Work out the finished part from the listing and answer in its coordinate system (mm). Face numbers are marked on the shaded views. Round coordinates to 2 decimals unless told otherwise and drop trailing zeros. Write each loop counter-clockwise with the first axis right and the second up, starting at its lowest first coordinate (ties: lowest second). Pieces come first, ordered by that corner, then holes. Notation, with made-up numbers: (-8.75, 42.5) -> (32.25, 42.5) arc R29 cw to (32.25, 77.5) -> close; hole circle Ø2 at (-35, -32.5). An arc over 180 degrees is marked (long way). One line per question, with ' | ' between items. Start each with the question number.
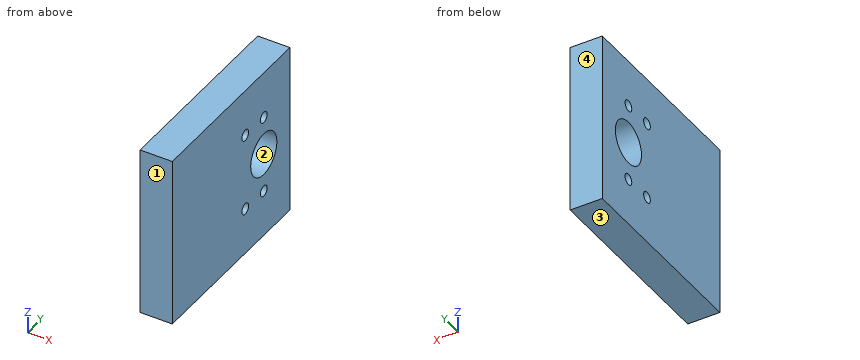
Autodesk Inventor part; units mm, degrees
ref_plane "YZ Plane" through (0, 0, 0) normal (1, 0, 0) x (0, 1, 0)
ref_plane "XZ Plane" through (0, 0, 0) normal (0, 1, 0) x (-1, 0, 0)
ref_plane "XY Plane" through (0, 0, 0) normal (0, 0, 1) x (1, 0, 0)
sketch "Sketch1" plane through (0, 0, 0) normal (1, 0, 0) x (0, 1, 0)
  line L0 (0, 0) -> (114.3, 0)
  line L1 (114.3, 0) -> (114.3, -101.6)
  line L2 (114.3, -101.6) -> (0, -101.6)
  line L3 (0, -101.6) -> (0, 0)
  dimension "d0" = 114.3
  dimension "d1" = 101.6
extrude "Extrusion1" add sketch "Sketch1" along normal blind 19.05
sketch "Sketch2" plane through (19.05, 0, 0) normal (1, 0, 0) x (0, 0, -1)
  circle A0 centre (27.8, 88.9) radius 3.2499
  circle A1 centre (73.8, 88.9) radius 3.2499
  circle A2 centre (73.8, 70.9) radius 3.2499
  circle A3 centre (27.8, 70.9) radius 3.2499
  line L0 (27.8, 88.9) -> (27.8, 70.9)
  line L1 (27.8, 88.9) -> (73.8, 88.9)
  line L2 (27.8, 70.9) -> (73.8, 70.9)
  line L3 (73.8, 70.9) -> (73.8, 88.9)
  line L4 (0, 114.3) -> (0, 0)
  line L5 (101.6, 0) -> (101.6, 114.3)
  line L6 (101.6, 114.3) -> (0, 114.3)
  dimension "d4" = 6.4999
  dimension "d5" = 6.4999
  dimension "d6" = 6.4999
  dimension "d7" = 6.4999
  dimension "d8" = 46
  dimension "d9" = 18
  dimension "d10" = 27.8
  dimension "d11" = 101.6
  dimension "d12" = 25.4
extrude "Extrusion2" cut sketch "Sketch2" against normal blind 19.05 contours L1 L0 A0 | A0 L0 L1 | L1 L3 A1 | A1 L3 L1 | L0 L2 A3 | A3 L2 L0 | L3 L2 A2 | A2 L2 L3
sketch "Sketch4" plane through (0, 0, 0) normal (-1, 0, 0) x (0, 0, 1)
  circle A0 centre (-50.8, 88.9) radius 12.7
  line L0 (-101.6, 114.3) -> (0, 114.3)
  circle A1 centre (-73.8, 88.9) radius 3.2499
  circle A2 centre (-27.8, 88.9) radius 3.2499
  line L1 (-73.8, 88.9) -> (-27.8, 88.9)
  point P0 (0, 0)
  dimension "d15" = 25.4
extrude "Extrusion3" cut sketch "Sketch4" against normal blind 19.05 contours L1 A0 | A0 L1
equation "\"d10\" = -0.5 * d8 + 0.5 * d11"
properties part number "X Axis Plate"
(1) Consider L1, parallel to Z at x = 11.25, y = 70.9; L2, parallel to Y at x = 4, z = -73.8; L3, parallel to Z at x = 7, y = 88.9. Determine where each line is inside the solid, lowest interval first.
(2) A cutting plane is placed at C-C, the plane z = -50.8. Determine the outline of the cut face in (x, y).
(3) A cutting plane is placed at B-B, the plane y = 88.9. Determine the outline of the cut face in (x, z), then the cut area to 3 significant figures.
(4) A cutting plane is placed at A-A, the plane y = 70.9. Determine the outline of the cut face in (x, z).
(5) A cutting plane is placed at D-D, the plane x = 14. Determine the outline of the cut face in (y, z).
(6) The mould has two halves that part along Y. Classify the marked faces 1, 2, 3 and 4: +Y half, -Y half, draft (parallel to the pull), parting line (faces both ways), or undercut.
(7) Given pin 1 Ø5 at (y, z) = (70.9, -27.8) entering from +X, flat-ended and moving along its own axis, determine where the tip first touches the part or whether it passes through.
Returned:
1) L1: -101.6 to -77.05, -70.55 to -31.05, -24.55 to 0 | L2: 0 to 67.65, 74.15 to 85.65, 92.15 to 114.3 | L3: -101.6 to -77.05, -70.55 to -63.5, -38.1 to -31.05, -24.55 to 0
2) outline: (0, 0) -> (19.05, 0) -> (19.05, 76.2) -> (0, 76.2) -> close; (0, 101.6) -> (19.05, 101.6) -> (19.05, 114.3) -> (0, 114.3) -> close
3) outline: (0, -101.6) -> (19.05, -101.6) -> (19.05, -77.05) -> (0, -77.05) -> close; (0, -70.55) -> (19.05, -70.55) -> (19.05, -63.5) -> (0, -63.5) -> close; (0, -38.1) -> (19.05, -38.1) -> (19.05, -31.05) -> (0, -31.05) -> close; (0, -24.55) -> (19.05, -24.55) -> (19.05, 0) -> (0, 0) -> close | area: 1,200 mm2
4) outline: (0, -101.6) -> (19.05, -101.6) -> (19.05, -77.05) -> (0, -77.05) -> close; (0, -70.55) -> (19.05, -70.55) -> (19.05, -31.05) -> (0, -31.05) -> close; (0, -24.55) -> (19.05, -24.55) -> (19.05, 0) -> (0, 0) -> close
5) outline: (0, -101.6) -> (114.3, -101.6) -> (114.3, 0) -> (0, 0) -> close; hole circle Ø6.5 at (70.9, -73.8); hole circle Ø6.5 at (70.9, -27.8); hole circle Ø25.4 at (88.9, -50.8); hole circle Ø6.5 at (88.9, -73.8); hole circle Ø6.5 at (88.9, -27.8)
6) face 1: -Y half | face 2: undercut | face 3: draft | face 4: +Y half
7) pin 1: through
